The listing builds one solid part. Answer for the finished solid, in the listing's coordinates (mm). Coordinates: 2 decimals unless noted, no trailing zeros. One line per question, with ' | ' between items.
from build123d import *

# Parameters (mm, degrees)
SKETCH_2_R          = 7.5
CUT_EXTRUDE_1_DEPTH = 8
SKETCH_3_RX         = 15
SKETCH_3_RY         = 7.5
CUT_EXTRUDE_2_DEPTH = 8
M3X0_51_D           = 2.5
M4X0_71_D           = 3.3
FILLET_1_R          = 1


with BuildPart() as part:
    # Эскиз1 → Повернуть1 (revolve)
    with BuildSketch(Plane.XY):
        Polygon((0, 0), (-43.5, 0), (-43.5, 3), (-30, 7), (0, 7), align=None)
    revolve(axis=Axis((0, 7, 0), (0, -1, 0)))

    # Эскиз2 → Вырез-Вытянуть1 (cut, through all)
    with BuildSketch(Plane(origin=(0, 7, 0), x_dir=(1, 0, 0), z_dir=(0, 1, 0))):
        Circle(SKETCH_2_R)
    extrude(amount=-CUT_EXTRUDE_1_DEPTH, mode=Mode.SUBTRACT)

    # Эскиз3 → Вырез-Вытянуть2 (cut, through all)
    with BuildSketch(Plane(origin=(0, 7, 0), x_dir=(1, 0, 0), z_dir=(0, 1, 0))):
        with Locations(Location((0, 35), (0, 0, -90))):
            Ellipse(SKETCH_3_RX, SKETCH_3_RY)
    extrude(amount=-CUT_EXTRUDE_2_DEPTH, mode=Mode.SUBTRACT)

    # Отверстие обработанное метчиком M3x0.51 (through all)
    with Locations(Plane(origin=(0, 7, 0), x_dir=(1, 0, 0), z_dir=(0, 1, 0))):
        with Locations((0, 15), (-15, 0), (0, -15), (15, 0)):
            Hole(M3X0_51_D / 2)

    # Отверстие обработанное метчиком M4x0.71 (through all)
    with Locations(Plane(origin=(0, 7, 0), x_dir=(1, 0, 0), z_dir=(0, 1, 0))):
        with Locations((-11.313708499, 11.313708499), (11.313708499, 11.313708499), (11.313708499, -11.313708499), (-11.313708499, -11.313708499)):
            Hole(M4X0_71_D / 2)

    # Скругление1
    fillet_1_edges = [part.edges().sort_by_distance(p)[0] for p in [
        (0, 7, 30),
        (0, 3, 43.5),
    ]]
    fillet(fillet_1_edges, radius=FILLET_1_R)


solid = part.part
Item 1: Section A-A, the plane x = 0 is taken. Count the separate pieces of the cut face and the enclosed holes in it, plus the area to 3 significant figures.
Computed values:
separate pieces: 4 | enclosed holes: 0 | area: 277 mm^2
Item 2: Find the intervals of material crossed by L1, parallel to Z at x = 0, y = 2; L2, parallel to X at y = 2.5, z = 14.5; L3, parallel to Z at x = -16, y = 2.25, in increasing order.
Computed values:
L1: z = -20 to -16.25, -13.75 to -7.5, 7.5 to 13.75, 16.25 to 43.5 | L2: x = -40.98 to -1.15, 1.15 to 40.98 | L3: z = -40.45 to -0.75, 0.75 to 40.45
Item 3: Determine the mould class of faces 1 (the face through (-1, 0, 9)), 2 (the face through (1.82, 1.14, 43.46)), 3 (the face through (16.25, 3.45, -0.05)) for opening direction X: pulls with the +X half, pulls with the -X half, needs draft (parallel to the pull), parting line crosses it, or undercut.
Computed values:
face 1: needs draft | face 2: parting line crosses it | face 3: undercut
Item 4: Each of these flat-tipped pins is pushed along its axis until it touches: pin 1 Ø8 at (x, z) = (-32.5, 28.5) entering from +Y; pin 2 Ø4 at (y, z) = (2.5, -15) entering from -X; pin 3 Ø2.5 at (x, z) = (11.31, -11.31) entering from -Y; pin 4 Ø12 at (x, z) = (-26, -31.5) entering from +Y. Where does it stop, or does it pass through?
Computed values:
pin 1: stops at y = 4.27 | pin 2: stops at x = -41.51 | pin 3: passes through | pin 4: stops at y = 5.56
